Part model, mm, in its own coordinate system. Round coordinates to 2 decimals unless told otherwise and drop trailing zeros. Write each loop counter-clockwise with the first axis right and the second up, starting at its lowest first coordinate (ties: lowest second). Pieces come first, ordered by that corner, then holes. Notation, with made-up numbers: M 67,67 L 74,67 A25 cw 74,85 Z; hole C -36,19.5 d8. An arc over 180 degrees is marked long. Use a Markdown table: item, result. Add a question column.
1) Wall check: probe 1 along Y at (x, z) = (64.5, 2.9); probe 2 along Y at (x, z) = (-98, 1.45); probe 3 along X at (y, z) = (-53, 2.3). Give the ranges that are in metal, low to high.
2) Slice it at A-A on y = -23.5. Write the cut outline in (x, z), plus the area to 3 significant figures.
3) Slice it at B-B on z = 1. Give the number of separate pieces and of enclosed holes in the cut face, plus the area to 3 significant figures.
4) Drop flat-ended pins along their axis: P1, Ø1, axis at y = 61, z = 1.5, coming from the +X side; P2, Ø3, axis at x = 97.75, y = 0, coming from the -Z side; P3, Ø1.6, axis at y = 57, z = 1, coming from the -X side; P4, Ø1, axis at x = 5.5, z = 1.5, coming from the -Y side. Give the stop position or say it passes through.
5) Slice it at C-C on y = 31. Write the cut outline in (x, z), plus the area to 3 significant figures.
```python
from build123d import *

# Parameters (mm, degrees)
SKETCH1_W               = 200
SKETCH1_H               = 125
BOSS_EXTRUDE1_DEPTH     = 3.18
SKETCH2_R               = 1.5
SKETCH2_W               = 3.18
SKETCH2_H               = 52.625
CUT_EXTRUDE1_DEPTH      = 4.18
SKETCH6_W               = 20
SKETCH6_H               = 3.18
CUT_EXTRUDE4_DEPTH      = 3.18
SKETCH7_W               = 32.709050062
SKETCH7_H               = 11.279604012
CUT_EXTRUDE5_DEPTH      = 3.18
SKETCH8_W               = 3.18
SKETCH8_H               = 19.75
CUT_EXTRUDE6_DEPTH      = 4.18
SKETCH9_W               = 3.18
SKETCH9_H               = 19.75
CUT_EXTRUDE7_DEPTH      = 4.18
SKETCH11_W              = 3.18
SKETCH11_H              = 20
BOSS_EXTRUDE3_DEPTH     = 3.18
CUT_EXTRUDE9_DEPTH      = 1
CUT_EXTRUDE9_DEPTH_BACK = 4.18
SKETCH13_W              = 3.18
SKETCH13_H              = 20
BOSS_EXTRUDE4_DEPTH     = 3.18
SKETCH14_R              = 1.59
CUT_EXTRUDE12_DEPTH     = 10


with BuildPart() as part:
    # Sketch1 → Boss-Extrude1 (new body)
    with BuildSketch(Plane.XY):
        Rectangle(SKETCH1_W, SKETCH1_H)
    extrude(amount=BOSS_EXTRUDE1_DEPTH)

    # Sketch2 → Cut-Extrude1 (cut, through all)
    with BuildSketch(Plane.XY.offset(3.18)):
        with Locations((-98, 0)):
            Circle(SKETCH2_R)
        with Locations((98, 0)):
            Circle(SKETCH2_R)
        Polygon((-10, 62.5), (10, 62.5), (10, 59.32), (1.5, 59.32), (1.5, 55.32), (3.5, 55.32), (3.5, 52.32), (1.5, 52.32), (1.5, 49.32), (-1.5, 49.32), (-1.5, 52.32), (-3.5, 52.32), (-3.5, 55.32), (-1.5, 55.32), (-1.5, 59.32), (-10, 59.32), align=None)
        Polygon((-10, -62.5), (-10, -59.32), (-1.5, -59.32), (-1.5, -55.32), (-3.5, -55.32), (-3.5, -52.32), (-1.5, -52.32), (-1.5, -49.32), (1.5, -49.32), (1.5, -52.32), (3.5, -52.32), (3.5, -55.32), (1.5, -55.32), (1.5, -59.32), (10, -59.32), (10, -62.5), align=None)
        with Locations((-98.41, 36.1875)):
            Rectangle(SKETCH2_W, SKETCH2_H)
        with Locations((-98.41, -36.1875)):
            Rectangle(SKETCH2_W, SKETCH2_H)
        with Locations((98.41, -36.1875)):
            Rectangle(SKETCH2_W, SKETCH2_H)
        with Locations((98.41, 36.1875)):
            Rectangle(SKETCH2_W, SKETCH2_H)
    extrude(amount=-CUT_EXTRUDE1_DEPTH, mode=Mode.SUBTRACT)

    # Sketch6 → Cut-Extrude4 (cut)
    with BuildSketch(Plane(origin=(0, 0, 0), x_dir=(-1, 0, 0), z_dir=(0, 0, -1))):
        with Locations((0, 4.478818731)):
            Rectangle(SKETCH6_W, SKETCH6_H)
    extrude(amount=-CUT_EXTRUDE4_DEPTH, mode=Mode.SUBTRACT)

    # Sketch7 → Cut-Extrude5 (cut)
    with BuildSketch(Plane(origin=(0, 0, 0), x_dir=(-1, 0, 0), z_dir=(0, 0, -1))):
        with Locations((-49.335490264, -26.125573068)):
            Rectangle(SKETCH7_W, SKETCH7_H)
    extrude(amount=-CUT_EXTRUDE5_DEPTH, mode=Mode.SUBTRACT)

    # Sketch8 → Cut-Extrude6 (cut, through all)
    with BuildSketch(Plane(origin=(0, 0, 0), x_dir=(-1, 0, 0), z_dir=(0, 0, -1))):
        with Locations((98.41, 0)):
            Rectangle(SKETCH8_W, SKETCH8_H)
    extrude(amount=-CUT_EXTRUDE6_DEPTH, mode=Mode.SUBTRACT)

    # Sketch9 → Cut-Extrude7 (cut, through all)
    with BuildSketch(Plane.XY.offset(3.18)):
        with Locations((98.41, 0)):
            Rectangle(SKETCH9_W, SKETCH9_H)
    extrude(amount=-CUT_EXTRUDE7_DEPTH, mode=Mode.SUBTRACT)

    # Sketch11 → Boss-Extrude3 (add, through all)
    with BuildSketch(Plane(origin=(0, 0, 0), x_dir=(-1, 0, 0), z_dir=(0, 0, -1))):
        with Locations((-98.41, 0)):
            Rectangle(SKETCH11_W, SKETCH11_H)
    extrude(amount=-BOSS_EXTRUDE3_DEPTH)

    # Sketch12 → Cut-Extrude9 (cut, two sides)
    with BuildSketch(Plane(origin=(0, 0, 0), x_dir=(-1, 0, 0), z_dir=(0, 0, -1))) as cut_extrude9_sk:
        with BuildLine():
            Line((-96.82, -0.926066952), (-96.82, 0.926066952))
            ThreePointArc((-96.82, 0.926066952), (-99.055723396, 0), (-96.82, -0.926066952))
        make_face()
    extrude(amount=CUT_EXTRUDE9_DEPTH, mode=Mode.SUBTRACT)
    extrude(cut_extrude9_sk.sketch, amount=-CUT_EXTRUDE9_DEPTH_BACK, mode=Mode.SUBTRACT)

    # Sketch13 → Boss-Extrude4 (add, through all)
    with BuildSketch(Plane(origin=(0, 0, 0), x_dir=(-1, 0, 0), z_dir=(0, 0, -1))):
        with Locations((98.41, 0)):
            Rectangle(SKETCH13_W, SKETCH13_H)
    extrude(amount=-BOSS_EXTRUDE4_DEPTH)

    # Sketch14 → Cut-Extrude12 (cut)
    with BuildSketch(Plane(origin=(0, 0, 0), x_dir=(-1, 0, 0), z_dir=(0, 0, -1))):
        with Locations((98, 0)):
            Circle(SKETCH14_R)
    extrude(amount=-CUT_EXTRUDE12_DEPTH, mode=Mode.SUBTRACT)


solid = part.part
```
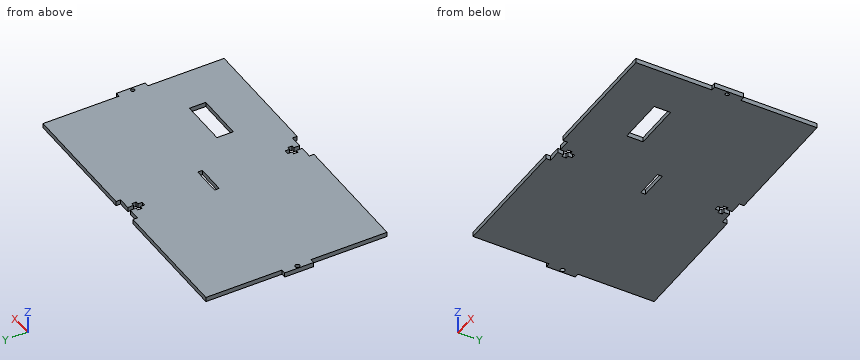
Entries:
| question | item | result |
|---|---|---|
| 1 | probe 1 | y = -62.5 to -31.77, -20.49 to 62.5 |
| 1 | probe 2 | y = -10 to -1.59, 1.59 to 10 |
| 1 | probe 3 | x = -96.82 to -3.5, 3.5 to 96.82 |
| 2 | outline | M -96.82,0 L 32.98,0 L 32.98,3.18 L -96.82,3.18 Z; M 65.69,0 L 96.82,0 L 96.82,3.18 L 65.69,3.18 Z |
| 2 | area | 512 mm^2 |
| 3 | separate pieces | 1 |
| 3 | enclosed holes | 4 |
| 3 | area | 23,700 mm^2 |
| 4 | P1 | stops at x = 96.82 |
| 4 | P2 | stops at z = 0 |
| 4 | P3 | stops at x = -96.82 |
| 4 | P4 | stops at y = -59.32 |
| 5 | outline | M -96.82,0 L 96.82,0 L 96.82,3.18 L -96.82,3.18 Z |
| 5 | area | 616 mm^2 |
